from build123d import *

# Parameters (mm, degrees)
IZIM1_R                     = 5
IZIM1_R_2                   = 3
Y_KSEKLIK_EKSTR_ZYON1_DEPTH = 150
IZIM2_R                     = 5
Y_KSEKLIK_EKSTR_ZYON2_DEPTH = 5
RADYUS1_R                   = 5


with BuildPart() as part:
    # Çizim1 → Yükseklik-Ekstrüzyon1 (new body)
    with BuildSketch(Plane(origin=(0, 0, 0), x_dir=(1, 0, 0), z_dir=(0, 1, 0))):
        with Locations(Location((0, 0, 0), (0, 0, 270))):
            Circle(IZIM1_R)
        with Locations(Location((0, 0, 0), (0, 0, 270))):
            Circle(IZIM1_R_2, mode=Mode.SUBTRACT)
    extrude(amount=Y_KSEKLIK_EKSTR_ZYON1_DEPTH)

    # Çizim2 → Yükseklik-Ekstrüzyon2 (add)
    with BuildSketch(Plane(origin=(0, 150, 0), x_dir=(1, 0, 0), z_dir=(0, 1, 0))):
        with Locations(Location((0, 0, 0), (0, 0, 270))):
            Circle(IZIM2_R)
    extrude(amount=Y_KSEKLIK_EKSTR_ZYON2_DEPTH)

    # Radyus1
    radyus1_edges = [part.edges().sort_by_distance(p)[0] for p in [
        (0, 155, -5),
    ]]
    fillet(radyus1_edges, radius=RADYUS1_R)


solid = part.part
The listing builds one solid part. Answer for the finished solid, in the listing's coordinates (mm). Give positions to 0.01 mm unless a question says otherwise; leave off trailing zeros. Write each loop counter-clockwise with the first axis right and the second up, starting at its lowest first coordinate (ties: lowest second). Pieces come first, ordered by that corner, then holes.
Item 1: Section A-A, the plane x = 0 is taken. Write down the section's boundary in (y, z), plus the area to 3 significant figures.
Item 2: Determine the mould class of faces 1 (the cylindrical face through (0.9, 73.95, 2.86)), 2 (the flat face through (-3.3, 0, -0.1)), 3 (the cylindrical face through (-4.88, 73.95, -1.08)) for opening direction Z: released by +Z, released by -Z, zero draft, split by the parting line, or undercut.
Item 3: Flat-ended cylindrical pins translate along their axes: P1, Ø3, axis at x = 0.5, z = -0.5, coming from the -Y side; P2, Ø5, axis at x = 3, y = 107.5, coming from the +Z side. Find the tip coordinate at first contact, or state that the pin passes through.
Item 4: Section B-B, the plane y = 81.5 is taken. Write down the section's boundary in (x, z), plus the area to 3 significant figures.
Item 5: Find the intervals of material crossed by line 1 along X through (y, z) = (67, 0); line 2 along Z through (x, y) = (-0.75, 30.5), in increasing order.
Item 6: Section C-C, the plane z = 0 is taken. Write down the section's boundary in (x, y), plus the area to 3 significant figures.
Completed:
1. outline: (0, -5) - (150, -5) arc R5 ccw to (150, 5) - (0, 5) - (0, 3) - (150, 3) - (150, -3) - (0, -3) - close
1. area: 639 mm2
2. face 1: undercut
2. face 2: zero draft
2. face 3: split by the parting line
3. P1: stops at y = 150
3. P2: stops at z = 4.97
4. outline: circle Ø10 at (0, 0); hole circle Ø6 at (0, 0)
4. area: 50.3 mm2
5. line 1: x = -5 to -3, 3 to 5
5. line 2: z = -4.94 to -2.9, 2.9 to 4.94
6. outline: (-5, 0) - (-3, 0) - (-3, 150) - (3, 150) - (3, 0) - (5, 0) - (5, 150) arc R5 ccw to (-5, 150) - close
6. area: 639 mm2
